Check sheet for the modelled part. Datum: model origin and axes. Units: mm. A direction names the side the tool comes from. Round coordinates to 2 decimals unless told otherwise and drop trailing zeros. Write each loop counter-clockwise with the first axis right and the second up, starting at its lowest first coordinate (ties: lowest second). Pieces come first, ordered by that corner, then holes. Notation, with made-up numbers: M 48.25,0.25 L 93.25,0.25 A13 ccw 93.25,23.25 Z; hole C 24.25,-32 d10. An arc over 180 degrees is marked long. Put each result on its own line as item: value.
```python
from build123d import *

# Parameters (mm, degrees)
SKETCH1_W           = 20
SKETCH1_H           = 35
SKETCH1_W_2         = 13
SKETCH1_H_2         = 23
BOSS_EXTRUDE1_DEPTH = 5
SKETCH2_R           = 1
CUT_EXTRUDE1_DEPTH  = 5
BOSS_EXTRUDE2_DEPTH = 5
FILLET1_R           = 2.5
SKETCH5_R           = 5
CUT_EXTRUDE2_DEPTH  = 5
SKETCH6_R           = 0.6
CUT_EXTRUDE3_DEPTH  = 5
CUT_EXTRUDE4_START  = -2.5
SKETCH8_R           = 0.6
SKETCH8_R_2         = 2.25
CUT_EXTRUDE4_DEPTH  = 2.5
FILLET2_R           = 2.5


with BuildPart() as part:
    # Sketch1 → Boss-Extrude1 (new body)
    with BuildSketch(Plane.XY):
        Rectangle(SKETCH1_W, SKETCH1_H)
        Rectangle(SKETCH1_W_2, SKETCH1_H_2, mode=Mode.SUBTRACT)
    extrude(amount=BOSS_EXTRUDE1_DEPTH)

    # Sketch2 → Cut-Extrude1 (cut)
    with BuildSketch(Plane.XY.offset(5)):
        with Locations((0, 13.9)):
            Circle(SKETCH2_R)
        with Locations(Location((0, -13.9, 0), (0, 0, 180))):
            Circle(SKETCH2_R)
    extrude(amount=-CUT_EXTRUDE1_DEPTH, mode=Mode.SUBTRACT)

    # Sketch3 → Boss-Extrude2 (add)
    with BuildSketch(Plane.ZY.offset(10)):
        Polygon((-5.5, 52.5), (-5.5, 17.5), (0, 17.5), (2.5, 17.5), (2.5, 52.5), align=None)
        Polygon((2.5, 52.5), (2.5, 17.5), (5, 17.5), (10.5, 17.5), (10.5, 52.5), align=None)
    extrude(amount=-BOSS_EXTRUDE2_DEPTH)

    # Fillet1
    fillet1_edges = [part.edges().sort_by_distance(p)[0] for p in [
        (-7.5, 17.5, 0),
        (-7.5, 17.5, 5),
    ]]
    fillet(fillet1_edges, radius=FILLET1_R)

    # Sketch5 → Cut-Extrude2 (cut)
    with BuildSketch(Plane(origin=(-5, 0, 0), x_dir=(0, 0, -1), z_dir=(1, 0, 0))):
        with Locations((-2.5, 42.5)):
            Circle(SKETCH5_R)
    extrude(amount=-CUT_EXTRUDE2_DEPTH, mode=Mode.SUBTRACT)

    # Sketch6 → Cut-Extrude3 (cut)
    with BuildSketch(Plane.ZY.offset(10)):
        with Locations((2.5, 38.05)):
            Circle(SKETCH6_R)
        with Locations((2.5, 36.05)):
            Circle(SKETCH6_R)
        with Locations((2.5, 34.05)):
            Circle(SKETCH6_R)
        with Locations((2.5, 32.05)):
            Circle(SKETCH6_R)
        with Locations((2.5, 30.05)):
            Circle(SKETCH6_R)
        with Locations((2.5, 28.05)):
            Circle(SKETCH6_R)
    extrude(amount=-CUT_EXTRUDE3_DEPTH, mode=Mode.SUBTRACT)

    # Sketch8 → Cut-Extrude4 (cut)
    # profile 1 of 4: a face of its own
    with BuildSketch(Plane.ZY.offset(10).offset(CUT_EXTRUDE4_START)):
        with BuildLine():
            ThreePointArc((2.245903559, 37.506460674), (-0.77838564, 38.72479304), (-2.408618858, 41.548442907))
            Line((-2.408618858, 41.548442907), (0.291121514, 27.621799308))
            ThreePointArc((0.291121514, 27.621799308), (0.594562485, 29.246581747), (1.926278936, 30.225625))
            ThreePointArc((1.926278936, 30.225625), (2.5, 30.65), (3.073721064, 30.225625))
            ThreePointArc((3.073721064, 30.225625), (4.282326064, 29.423249359), (4.75, 28.05))
            ThreePointArc((4.75, 28.05), (4.739696028, 27.834914661), (4.708878486, 27.621799308))
            Line((4.708878486, 27.621799308), (7.408618858, 41.548442907))
            ThreePointArc((7.408618858, 41.548442907), (5.77838564, 38.72479304), (2.754096441, 37.506460674))
            ThreePointArc((2.754096441, 37.506460674), (2.5, 37.45), (2.245903559, 37.506460674))
        make_face()
        with Locations((2.5, 32.05)):
            Circle(SKETCH8_R, mode=Mode.SUBTRACT)
        with Locations((2.5, 34.05)):
            Circle(SKETCH8_R, mode=Mode.SUBTRACT)
        with Locations((2.5, 36.05)):
            Circle(SKETCH8_R, mode=Mode.SUBTRACT)
    # profile 2 of 4: a face of its own
    with BuildSketch(Plane.ZY.offset(10).offset(CUT_EXTRUDE4_START)):
        with Locations((2.5, 28.05)):
            Circle(SKETCH8_R_2)
        with Locations((2.5, 28.05)):
            Circle(SKETCH8_R, mode=Mode.SUBTRACT)
    # profile 3 of 4: a face of its own
    with BuildSketch(Plane.ZY.offset(10).offset(CUT_EXTRUDE4_START)):
        with Locations((2.5, 30.05)):
            Circle(SKETCH8_R)
    # profile 4 of 4: a face of its own
    with BuildSketch(Plane.ZY.offset(10).offset(CUT_EXTRUDE4_START)):
        with BuildLine():
            ThreePointArc((7.5, 42.5), (2.022032581, 47.477102284), (-2.408618858, 41.548442907))
            ThreePointArc((-2.408618858, 41.548442907), (-0.77838564, 38.72479304), (2.245903559, 37.506460674))
            ThreePointArc((2.245903559, 37.506460674), (2.5, 37.5), (2.754096441, 37.506460674))
            ThreePointArc((2.754096441, 37.506460674), (5.77838564, 38.72479304), (7.408618858, 41.548442907))
            ThreePointArc((7.408618858, 41.548442907), (7.477102284, 42.022032581), (7.5, 42.5))
        make_face()
    extrude(amount=CUT_EXTRUDE4_DEPTH, mode=Mode.SUBTRACT)

    # Fillet2
    fillet2_edges = [part.edges().sort_by_distance(p)[0] for p in [
        (-10, -17.5, 2.5),
        (-5, 17.5, 2.5),
        (10, 17.5, 2.5),
        (10, -17.5, 2.5),
        (-7.5, 17.5, 10.5),
        (-7.5, 52.5, 10.5),
        (-7.5, 52.5, -5.5),
        (-7.5, 17.5, -5.5),
    ]]
    fillet(fillet2_edges, radius=FILLET2_R)


solid = part.part
```
1. Cross-section at B-B (y = -5). Enter the section's corners in (x, z), then the cut area to 3 significant figures.
Computed values:
outline: M -10,0 L -6.5,0 L -6.5,5 L -10,5 Z; M 6.5,0 L 10,0 L 10,5 L 6.5,5 Z
area: 35.0 mm2
2. Cross-section at C-C (z = -1.25). Enter the section's corners in (x, y).
Computed values:
outline: M -10,17.17 L -5,17.17 L -5,39.19 L -7.5,39.19 L -7.5,35.57 L -10,35.57 Z; M -10,45.81 L -5,45.81 L -5,52.5 L -10,52.5 Z
3. Depth check by flat-ended pin: pin 1 Ø1.6 at (y, z) = (30.05, 2.5) entering from +X; pin 2 Ø1 at (y, z) = (-5, -1) entering from +X; pin 3 Ø6 at (x, y) = (-4, 10.5) entering from +Z; pin 4 Ø1.4 at (y, z) = (34.05, 2.5) entering from -X. Enter the tip coordinate at first touch or a pass-through.
Computed values:
pin 1: stops at x = -5
pin 2: passes through
pin 3: stops at z = 5
pin 4: stops at x = -7.5
4. Access from +Z, -Z, +X, -X, +Y, -Y to the whole of each face (thin tool, end or side, straight path). Record for faces 1 (the flat face through (-8, 35, -5.5)), 2 (the flat face through (0, -11.5, 2)), 3 (the flat face through (-8.73, 34.49, 6.04)).
Computed values:
face 1: -Z, +X, -X, +Y, -Y
face 2: +Z, -Z
face 3: -X
5. Cross-section at A-A (x = 0). Enter the section's corners in (y, z), then the cut area to 3 significant figures.
Computed values:
outline: M -17.5,0 L -14.9,0 L -14.9,5 L -17.5,5 Z; M -12.9,0 L -11.5,0 L -11.5,5 L -12.9,5 Z; M 11.5,0 L 12.9,0 L 12.9,5 L 11.5,5 Z; M 14.9,0 L 17.5,0 L 17.5,5 L 14.9,5 Z
area: 40.0 mm2
6. Scan lines: probe 1 along Y at (x, z) = (0, 2.7); probe 2 along X at (y, z) = (6, 0.5); probe 3 along Y at (x, z) = (1.25, 3.75). Record each from-to range of solid material in increasing order.
Computed values:
probe 1: y = -17.5 to -14.9, -12.9 to -11.5, 11.5 to 12.9, 14.9 to 17.5
probe 2: x = -10 to -6.5, 6.5 to 10
probe 3: y = -17.5 to -11.5, 11.5 to 17.5
7. Release check for a two-part mould opening along Z. For faces 4 (the cylindrical face through (-6.268, 29.464, 2.37)), 5 (the flat face through (-8.732, 34.683, -1.078)), 6 (the cylindrical face through (-7.465, 18.252, 9.787)), 7 (the flat face through (0, 11.5, 2)) record: +Z half, -Z half, draft (parallel to the pull), parting line (faces both ways), or undercut.
Computed values:
face 4: undercut
face 5: undercut
face 6: +Z half
face 7: draft
8. Cross-section at D-D (y = 42.5). Enter the section's corners in (x, z).
Computed values:
outline: M -10,-5.5 L -5,-5.5 L -5,-2.5 L -10,-2.5 Z; M -10,7.5 L -5,7.5 L -5,10.5 L -10,10.5 Z
